Autodesk Inventor part; units mm, degrees
ref_plane "YZ Plane" through (0, 0, 0) normal (1, 0, 0) x (0, 1, 0)
ref_plane "XZ Plane" through (0, 0, 0) normal (0, 1, 0) x (-1, 0, 0)
ref_plane "XY Plane" through (0, 0, 0) normal (0, 0, 1) x (1, 0, 0)
sketch "Sketch1" plane through (0, 0, 0) normal (0, 0, 1) x (1, 0, 0)
  line L0 (0, 0) -> (10, 0)
  line L1 (10, 0) -> (10, 48)
  line L2 (10, 48) -> (0, 48)
  circle A0 centre (-2, 7.5) radius 4
  arc A1 (0, 27.8586) -> (0, 42.1414) centre (-7, 35) ccw
  line L3 (-2, 11.5) -> (0, 11.5)
  line L4 (0, 11.5) -> (0, 3.5)
  line L5 (0, 3.5) -> (-2, 3.5)
  line L6 (-2, 3.5) -> (-2, 11.5)
  line L7 (0, 48) -> (0, 42.1414)
  line L8 (0, 27.8586) -> (0, 0)
  dimension "d90" = 8
  dimension "d0" = 10
  dimension "d1" = 48
  dimension "d88" = 12
  dimension "d89" = 7.5
  dimension "d91" = 20
  dimension "d92" = 13
extrude "Extrusion1" add sketch "Sketch1" along normal blind 3
fillet "圓角5" radius 2 8 edges at (0, 0, 1.5) (0, 3.5, 1.5) (0, 11.5, 1.5) (10, 0, 1.5) (0, 27.8586, 1.5) (0, 42.1414, 1.5) (0, 48, 1.5) (10, 48, 1.5)
sketch "草圖9" plane through (0, 0, 3) normal (0, 0, 1) x (1, 0, 0)
  line L0 (2, 48) -> (8, 48)
  arc A0 (-2, 11.5) -> (-2, 3.5) centre (-2, 7.5) ccw
  line L1 (8, 0) -> (2, 0)
  line L2 (10, 46) -> (10, 2)
  point P0 (0, 0)
  point P1 (4, 24.5)
  point P2 (5, 41)
  dimension "d95" = 6
  dimension "d96" = 24.5
  dimension "d97" = 7
  dimension "d98" = 5
hole "孔5" at (-2, 7.5, 3) at (4, 24.5, 3) at (5, 41, 3) direction (0, 0, -1) diameter 3 end through all
properties part number "plastic_part_53"
The listing builds one solid part. Answer for the finished solid, in the listing's coordinates (mm). A direction names the side the tool comes from. Round coordinates to 2 decimals unless told otherwise and drop trailing zeros. Order: outer loops, then holes, each group sorted by start corner. A loop starts at its lowest first (then second) coordinate and runs counter-clockwise, first axis right, second up. Notation, with made-up numbers: M -20.75,-18 L 18.25,-18 A29 ccw 18.25,13 Z; hole C 28,-12.5 d7. An arc over 180 degrees is marked long. Answer in a Markdown table with one row per item. Add a question column.
1) Flat-ended cylindrical pins translate along their axes: pin 1 Ø1.5 at (y, z) = (19, 1) entering from -X; pin 2 Ø1.8 at (x, y) = (5, 41) entering from +Z. Find the tip coordinate at first contact, or state that the pin passes through.
2) Determine the mould class of faces 1 (the face through (0, 44, 1)), 2 (the face through (5, 0, 1)), 3 (the face through (4, 26, 1)) for opening direction X: pulls with the +X half, pulls with the -X half, needs draft (parallel to the pull), parting line crosses it, or undercut.
3) The part is cut by section B-B on x = 4. Determine the outline of the cut face in (y, z), plus the area to 3 significant figures.
4) Consider line 1 along Y through (x, z) = (5, 1.95); line 2 along X through (y, z) = (24.5, 1.55); line 3 along Y through (x, z) = (4.25, 0.4). Determine where each line is inside the solid, lowest interval first. Write a range as from..to.
5) Which of the six approach directions +Z, -Z, +X, -X, +Y, -Y give full straight-line access (tool end or side, diameter ignored) to faces 4 (the face through (4.93, 42.5, 1.48)), 5 (the face through (0.133, 27.779, 1.521)), 6 (the face through (0, 20, 1))?
6) The part is cut by section C-C on z = 1.2. Count the separate pieces of the cut face and the enclosed holes in it, plus the area to 3 significant figures.
7) The part is cut by section A-A on y = 7.5. Determine the outline of the cut face in (x, z), plus the area to 3 significant figures.
8) The part is cut by section D-D on y = 24.5. Determine the outline of the cut face in (x, z).
Findings below:
| question | item | result |
|---|---|---|
| 1 | pin 1 | stops at x = 0 |
| 1 | pin 2 | passes through |
| 2 | face 1 | pulls with the -X half |
| 2 | face 2 | needs draft |
| 2 | face 3 | undercut |
| 3 | outline | M 0,0 L 23,0 L 23,3 L 0,3 Z; M 26,0 L 39.88,0 L 39.88,3 L 26,3 Z; M 42.12,0 L 48,0 L 48,3 L 42.12,3 Z |
| 3 | area | 128 mm² |
| 4 | line 1 | y = 0..23.38, 25.62..39.5, 42.5..48 |
| 4 | line 2 | x = 0..2.5, 5.5..10 |
| 4 | line 3 | y = 0..23.02, 25.98..39.7, 42.3..48 |
| 5 | face 4 | +Z, -Z |
| 5 | face 5 | +Z, -Z, -X |
| 5 | face 6 | +Z, -Z, -X, +Y |
| 6 | separate pieces | 1 |
| 6 | enclosed holes | 3 |
| 6 | area | 468 mm² |
| 7 | outline | M -6,0 L -3.5,0 L -3.5,3 L -6,3 Z; M -0.5,0 L 10,0 L 10,3 L -0.5,3 Z |
| 7 | area | 39.0 mm² |
| 8 | outline | M 0,0 L 2.5,0 L 2.5,3 L 0,3 Z; M 5.5,0 L 10,0 L 10,3 L 5.5,3 Z |
